Could you check a few things on this model? Use its own coordinates, in mm. A direction names the side the tool comes from. Round coordinates to 2 decimals unless told otherwise and drop trailing zeros. Loops run counter-clockwise (first coordinate to the right, second up) from the corner with the lowest first, then second, coordinate; pieces in that order, holes last. Notation, with made-up numbers: (49.5, 69.25) -> (88.5, 69.25) arc R11 cw to (88.5, 86.25) -> close; hole circle Ø2 at (61.25, -14). An arc over 180 degrees is marked (long way). One line per item, written item: value.
from build123d import *

# Parameters (mm, degrees)
Y_KSEKLIK_EKSTR_ZYON1_DEPTH = 25
IZIM4_R                     = 2.6
KES_EKSTR_ZYON1_DEPTH       = 9
IZIM5_R                     = 4.6
KES_EKSTR_ZYON2_DEPTH       = 6
IZIM6_R                     = 2.6
KES_EKSTR_ZYON3_DEPTH       = 36.5
IZIM7_R                     = 4.6
KES_EKSTR_ZYON4_DEPTH       = 5
RADYUS1_R                   = 0.5


with BuildPart() as part:
    # Çizim1 → Yükseklik-Ekstrüzyon1 (new body)
    with BuildSketch(Plane.XY):
        with BuildLine():
            Line((6.516322935, -38.083207178), (6.516322935, -24.224071188))
            ThreePointArc((6.516322935, -24.224071188), (6.839093945, -23.488298875), (7.599044726, -23.227498508))
            ThreePointArc((7.599044726, -23.227498508), (19.398597482, -13.819653137), (10.702548541, -1.486132448))
            ThreePointArc((10.702548541, -1.486132448), (10.303139514, -1.025885698), (10.645127383, -0.521505941))
            Line((10.645127383, -0.521505941), (32.763677784, 6.800349322))
            ThreePointArc((32.763677784, 6.800349322), (33.527004842, 6.744508119), (34.027272888, 6.165268687))
            Line((34.027272888, 6.165268687), (34.655787357, 4.266592948))
            ThreePointArc((34.655787357, 4.266592948), (34.599946154, 3.50326589), (34.020706721, 3.002997844))
            Line((34.020706721, 3.002997844), (29.970072893, 1.662125405))
            ThreePointArc((29.970072893, 1.662125405), (24.517159095, -2.720713399), (23.271180913, -9.604831589))
            ThreePointArc((23.271180913, -9.604831589), (22.043278837, -18.732259795), (15.713387532, -25.421816227))
            ThreePointArc((15.713387532, -25.421816227), (11.913144626, -29.095314243), (10.516322935, -34.192894354))
            Line((10.516322935, -34.192894354), (10.516322935, -38.083207178))
            ThreePointArc((10.516322935, -38.083207178), (10.223429716, -38.790313959), (9.516322935, -39.083207178))
            Line((9.516322935, -39.083207178), (7.516322935, -39.083207178))
            ThreePointArc((7.516322935, -39.083207178), (6.809216154, -38.790313959), (6.516322935, -38.083207178))
        make_face()
    extrude(amount=-Y_KSEKLIK_EKSTR_ZYON1_DEPTH)

    # Çizim4 → Kes-Ekstrüzyon1 (cut)
    with BuildSketch(Plane(origin=(15.516322935, 0, 0), x_dir=(0, 0, -1), z_dir=(1, 0, 0))):
        with Locations((12.5, -29.783207178)):
            Circle(IZIM4_R)
    extrude(amount=-KES_EKSTR_ZYON1_DEPTH, mode=Mode.SUBTRACT)

    # Çizim5 → Kes-Ekstrüzyon2 (cut)
    with BuildSketch(Plane(origin=(15.516322935, 0, 0), x_dir=(0, 0, -1), z_dir=(1, 0, 0))):
        with Locations((12.5, -29.783207178)):
            Circle(IZIM5_R)
    extrude(amount=-KES_EKSTR_ZYON2_DEPTH, mode=Mode.SUBTRACT)

    # Çizim6 → Kes-Ekstrüzyon3 (cut)
    with BuildSketch(Plane(origin=(20.440424649, -15.226956818, 0), x_dir=(0, 0, 1), z_dir=(0.801942288, -0.597401512, 0))):
        with Locations((-12.5, -14.66586446)):
            Circle(IZIM6_R)
    extrude(amount=-KES_EKSTR_ZYON3_DEPTH, mode=Mode.SUBTRACT)

    # Çizim7 → Kes-Ekstrüzyon4 (cut)
    with BuildSketch(Plane(origin=(20.440424649, -15.226956818, 0), x_dir=(0, 0, 1), z_dir=(0.801942288, -0.597401512, 0))):
        with Locations((-12.5, -14.66586446)):
            Circle(IZIM7_R)
    extrude(amount=-KES_EKSTR_ZYON4_DEPTH, mode=Mode.SUBTRACT)

    # Radyus1
    radyus1_edges = [part.edges().sort_by_distance(p)[0] for p in [
        (24.517159095, -2.720713399, -25),
        (10.516322935, -36.138050766, 0),
        (10.223429716, -38.790313959, 0),
        (8.516322935, -39.083207178, 0),
        (31.995389807, 2.332561624, -25),
        (6.809216154, -38.790313959, 0),
        (6.516322935, -31.153639183, 0),
        (6.839093945, -23.488298875, 0),
        (19.398597482, -13.819653137, 0),
        (10.303139514, -1.025885698, 0),
        (21.704402584, 3.13942169, 0),
        (33.527004842, 6.744508119, 0),
        (34.341530122, 5.215930817, 0),
        (34.599946154, 3.50326589, 0),
        (31.995389807, 2.332561624, 0),
        (34.599946154, 3.50326589, -25),
        (24.517159095, -2.720713399, 0),
        (22.043278837, -18.732259795, 0),
        (11.913144626, -29.095314243, 0),
        (34.341530122, 5.215930817, -25),
        (33.527004842, 6.744508119, -25),
        (21.704402584, 3.13942169, -25),
        (10.303139514, -1.025885698, -25),
        (19.398597482, -13.819653137, -25),
        (6.839093945, -23.488298875, -25),
        (6.516322935, -31.153639183, -25),
        (11.913144626, -29.095314243, -25),
        (6.809216154, -38.790313959, -25),
        (8.516322935, -39.083207178, -25),
        (10.223429716, -38.790313959, -25),
        (10.516322935, -36.138050766, -25),
        (22.043278837, -18.732259795, -25),
    ]]
    fillet(radyus1_edges, radius=RADYUS1_R)


solid = part.part
(1) If we section it at A-A, the plane z = -12.5: Give the number of separate pieces and of enclosed holes in the cut face, then the cut area to 3 significant figures.
Recorded:
separate pieces: 3
enclosed holes: 0
area: 224 mm²
(2) I'm going to push flat-ended pins straight in: pin 1 Ø1 at (x, z) = (18.5, -14) entering from -Y; pin 2 Ø3 at (y, z) = (-30.5, -14) entering from +X; pin 3 Ø4 at (y, z) = (-29.78, -12.5) entering from +X; pin 4 Ø3 at (x, z) = (26.5, -8) entering from +Y. Where does each tip first touch, or does it pass through?
Recorded:
pin 1: y = -23.88
pin 2: x = 9.52
pin 3: through
pin 4: y = 5.22
(3) For faces 5 (the face through (21.906, 3.048, -24.857)), 6 (the face through (11.892, -25.222, -11.901)), which set-ups out of +Z, -Z, +X, -X, +Y, -Y let a thin tool reach every point of the face, with its end or its side?
Recorded:
face 5: -Z, -X, +Y
face 6: none
(4) If we section it at B-B, the plane z = -4.25: Please give me the cut outline in (x, y).
Recorded:
outline: (6.52, -38.08) arc R1 ccw to (7.52, -39.08) -> (9.52, -39.08) arc R1 ccw to (10.52, -38.08) -> (10.52, -34.19) arc R10 cw to (15.71, -25.42) arc R15 ccw to (23.27, -9.6) arc R10 cw to (29.97, 1.66) -> (34.02, 3) arc R1 ccw to (34.66, 4.27) -> (34.03, 6.17) arc R1 ccw to (32.76, 6.8) -> (10.65, -0.52) arc R0.5 ccw to (10.7, -1.49) arc R11 cw to (7.6, -23.23) arc R1 ccw to (6.52, -24.22) -> close
(5) Thinking about a two-plate mould opening in Y: for faces 1 (the face through (31.92, 2.47, -0.14)), 2 (the face through (19.363, -14.05, -12.332)), 3 (the face through (34.2, 5.16, -24.86)), 4 (the face through (10.516, -36, -12)), which applies, released by +Y, released by -Y, zero draft, split by the parting line, or undercut?
Recorded:
face 1: released by -Y
face 2: undercut
face 3: released by +Y
face 4: zero draft
(6) If I drill on L1, parallel to Y at x = 8.2, z = -12.5; L2, parallel to X at y = -34.5, z = -10; L3, parallel to Y at x = 12.75, z = -12.5, over which ranges is the centre line in solid material (lowest first)?
Recorded:
L1: -39.08 to -32.38, -27.18 to -23.26
L2: 6.52 to 10.52
L3: -25.18 to -22.41, -2.12 to 0.18
